Work out the finished part from the listing and answer in its coordinate system (mm). Give positions to 0.01 mm unless a question says otherwise; leave off trailing zeros. Order: outer loops, then holes, each group sorted by start corner. A loop starts at its lowest first (then second) coordinate and runs counter-clockwise, first axis right, second up. Notation, with made-up numbers: M 3,54 L 45,54 A29 cw 45,85 Z; hole C 51,62.5 d6. An arc over 180 degrees is marked long. One line per item, written item: value.
from build123d import *

# Parameters (mm, degrees)
BOSS_EXTRUDE1_DEPTH       = 3.175
SKETCH2_W                 = 1.5875
SKETCH2_H                 = 3.175
CUT_EXTRUDE1_DEPTH        = 3.175
F_2_56_TAPPED_HOLE1_D     = 1.778
F_2_56_TAPPED_HOLE1_DEPTH = 5.588
F_2_56_TAPPED_HOLE1_TIP   = 0.53416509
F_2_56_TAPPED_HOLE2_D     = 1.778
F_2_56_TAPPED_HOLE2_DEPTH = 10.668
F_2_56_TAPPED_HOLE2_TIP   = 0.53416509
F_2_56_TAPPED_HOLE3_D     = 1.778
F_2_56_TAPPED_HOLE3_DEPTH = 10.668
F_2_56_TAPPED_HOLE3_TIP   = 0.53416509


with BuildPart() as part:
    # Sketch1 → Boss-Extrude1 (new body, symmetric)
    with BuildSketch(Plane(origin=(0, 0, 0), x_dir=(0, 0, -1), z_dir=(1, 0, 0))):
        Polygon((-6.35, -6.892849115), (-44.45, -6.892849115), (-44.45, 2.632150885), (82.55, 2.632150885), (82.55, -6.892849115), (6.35, -6.892849115), (6.35, -29.117849115), (-6.35, -29.117849115), align=None)
    extrude(amount=BOSS_EXTRUDE1_DEPTH, both=True)

    # Sketch2 → Cut-Extrude1 (cut)
    with BuildSketch(Plane(origin=(0, 0, -6.35), x_dir=(-1, 0, 0), z_dir=(0, 0, -1))):
        with Locations((-0.79375, -11.072771518)):
            Rectangle(SKETCH2_W, SKETCH2_H)
        with Locations((-0.79375, -23.772771518)):
            Rectangle(SKETCH2_W, SKETCH2_H)
    extrude(amount=-CUT_EXTRUDE1_DEPTH, mode=Mode.SUBTRACT)

    # #2-56 Tapped Hole1
    with Locations(Plane(origin=(3.175, 0, 0), x_dir=(0, 0, -1), z_dir=(1, 0, 0))):
        with Locations((-3.175, -6.892849115)):
            Hole(F_2_56_TAPPED_HOLE1_D / 2, depth=F_2_56_TAPPED_HOLE1_DEPTH)
            with Locations((0, 0, -(F_2_56_TAPPED_HOLE1_DEPTH + F_2_56_TAPPED_HOLE1_TIP / 2))):  # 118° drill point
                Cone(0, F_2_56_TAPPED_HOLE1_D / 2, F_2_56_TAPPED_HOLE1_TIP, mode=Mode.SUBTRACT)

    # #2-56 Tapped Hole2
    with Locations(Plane.XY.offset(44.45)):
        with Locations((0, -2.130349115)):
            Hole(F_2_56_TAPPED_HOLE2_D / 2, depth=F_2_56_TAPPED_HOLE2_DEPTH)
            with Locations((0, 0, -(F_2_56_TAPPED_HOLE2_DEPTH + F_2_56_TAPPED_HOLE2_TIP / 2))):  # 118° drill point
                Cone(0, F_2_56_TAPPED_HOLE2_D / 2, F_2_56_TAPPED_HOLE2_TIP, mode=Mode.SUBTRACT)

    # #2-56 Tapped Hole3
    with Locations(Plane(origin=(0, 0, -82.55), x_dir=(-1, 0, 0), z_dir=(0, 0, -1))):
        with Locations((0, -2.130349115)):
            Hole(F_2_56_TAPPED_HOLE3_D / 2, depth=F_2_56_TAPPED_HOLE3_DEPTH)
            with Locations((0, 0, -(F_2_56_TAPPED_HOLE3_DEPTH + F_2_56_TAPPED_HOLE3_TIP / 2))):  # 118° drill point
                Cone(0, F_2_56_TAPPED_HOLE3_D / 2, F_2_56_TAPPED_HOLE3_TIP, mode=Mode.SUBTRACT)


solid = part.part
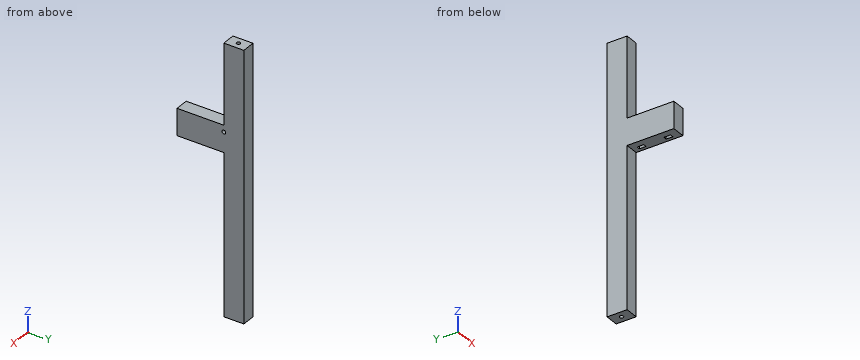
(1) Section A-A, the plane z = -73 is taken. Give the vertices of the cut face in (x, y) (3 decimals).
Findings:
outline: M -3.175,-6.893 L 3.175,-6.893 L 3.175,2.632 L -3.175,2.632 Z; hole C 0,-2.13 d1.778
(2) Section B-B, the plane y = -17 is taken. Give the vertices of the cut face in (x, z) (3 decimals), then the cut area to 3 significant figures.
Findings:
outline: M -3.175,-6.35 L 3.175,-6.35 L 3.175,6.35 L -3.175,6.35 Z
area: 80.6 mm^2
(3) Section C-C, the plane z = -20 is taken. Give the vertices of the cut face in (x, y) (3 decimals), then the cut area to 3 significant figures.
Findings:
outline: M -3.175,-6.893 L 3.175,-6.893 L 3.175,2.632 L -3.175,2.632 Z
area: 60.5 mm^2
(4) Find the intervals of material crossed by probe 1 along Y at (x, z) = (0, 39.25); probe 2 along Z at (x, y) = (0.75, -7); probe 3 along Z at (x, y) = (-0.75, -22.5), in increasing order. Write a range as from..to.
Findings:
probe 1: y = -6.89..-3.02, -1.24..2.63
probe 2: z = -6.35..2.29, 4.06..6.35
probe 3: z = -6.35..6.35
(5) Given P1, Ø1.5, axis at x = 1, z = 15.5, coming from the -Y side; P2, Ø3, axis at x = 0.5, y = -22, coming from the +Z side; P3, Ø1.6, axis at y = -6.89, z = 3.18, coming from the +X side, each flat-ended and moving along its own axis, determine where each tip first touches the part or whether it passes through.
Findings:
P1: stops at y = -6.89
P2: stops at z = 6.35
P3: stops at x = -2.46
